For this review, use the dimensioned drawing (mm, ordinates from the lowest corner) and the shaded views. A direction names the side the tool comes from. Coordinates: 2 decimals unless noted, no trailing zeros. Loops run counter-clockwise (first coordinate to the right, second up) from the corner with the lowest first, then second, coordinate; pieces in that order, holes last. Notation, with made-up numbers: (1, 13.25) - (26, 13.25) arc R14 ccw to (26, 18.25) - close; hole circle Ø6 at (89.25, 78.5). An arc over 180 degrees is marked (long way). Answer in a Markdown table with one row per item. Add a question column.
(1) Machinability: for the marked faces 5 and 6, which of the approach directions +Z, -Z, +X, -X, +Y, -Y give a long, thin tool a straight path to every point of the face, cutting with its end or side? Answer none if there is none.
(2) We need section D-D on y = 1.5. Write out the cut boundary in (x, z), plus the area to 3 significant figures.
(3) We need section C-C on z = 4.75. Write out the cut boundary in (x, y).
(4) For line 1 along X through (y, z) = (2.75, 2.5) (3 decimals); line 2 along X through (y, z) = (4.5, 3.25); line 3 along Y through (x, z) = (6, 6), list the stretches that pass through material, from the lowest coordinate up.
(5) We need section A-A on y = 5.5. Write out the cut boundary in (x, z).
(6) For P1, Ø1.5, axis at y = 2.5, z = 2, coming from the +X side; P2, Ø3, axis at x = 20, z = 4, coming from the +Y side; P3, Ø1.5, axis at y = 6.5, z = 3.5, coming from the +X side; P4, Ø4, axis at x = 24, z = 3, coming from the +Y side, all flat-tipped, find the tip position at first contact; note any pin that passes through.
(7) Mouldability with a two-part tool opening along X and no side actions: class the marked faces 1, 2, 3 and 4 as +X half, -X half, draft (parallel to the pull), parting line (faces both ways), or undercut.
(8) We need section B-B on x = 20. Write out the cut boundary in (y, z).
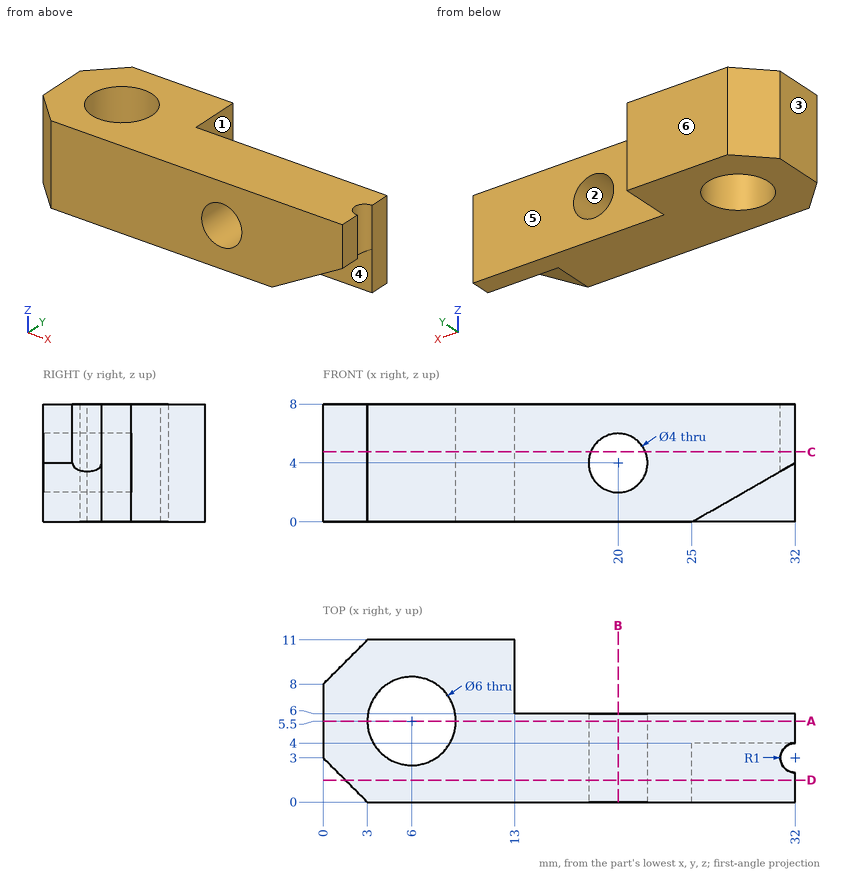
Outcome:
| question | item | result |
|---|---|---|
| 1 | face 5 | +Z, -Z, +X, +Y |
| 1 | face 6 | +Z, -Z, +X, -X, +Y |
| 2 | outline | (1.5, 0) - (25, 0) - (32, 4) - (32, 8) - (1.5, 8) - close; hole circle Ø4 at (20, 4) |
| 2 | area | 217 mm² |
| 3 | outline | (0, 3) - (3, 0) - (18.15, 0) - (18.15, 6) - (13, 6) - (13, 11) - (3, 11) - (0, 8) - close; (21.85, 0) - (32, 0) - (32, 2) arc R1 cw to (32, 4) - (32, 6) - (21.85, 6) - close; hole circle Ø6 at (6, 5.5) |
| 4 | line 1 | 0.25 to 4.801, 7.199 to 18.677, 21.323 to 29.375 |
| 4 | line 2 | 0 to 3.17, 8.83 to 18.15, 21.85 to 32 |
| 4 | line 3 | 0 to 2.5, 8.5 to 11 |
| 5 | outline | (0, 0) - (3, 0) - (3, 8) - (0, 8) - close; (9, 0) - (32, 0) - (32, 8) - (9, 8) - close; hole circle Ø4 at (20, 4) |
| 6 | P1 | x = 29.81 |
| 6 | P2 | through |
| 6 | P3 | x = 32 |
| 6 | P4 | y = 6 |
| 7 | face 1 | +X half |
| 7 | face 2 | undercut |
| 7 | face 3 | -X half |
| 7 | face 4 | draft |
| 8 | outline | (0, 0) - (6, 0) - (6, 2) - (0, 2) - close; (0, 6) - (6, 6) - (6, 8) - (0, 8) - close |
